Build history of the part. All positions in model axes, mm. Give positions to 0.01 mm unless a question says otherwise; leave off trailing zeros. Order: outer loops, then holes, each group sorted by start corner. A loop starts at its lowest first (then second) coordinate and runs counter-clockwise, first axis right, second up. Notation, with made-up numbers: (39.5, 25) -> (49.5, 25) arc R8 ccw to (49.5, 40) -> close; hole circle Ø8 at (42, -34.75). An arc over 180 degrees is marked (long way). One line per item, written item: value. Start each with the question number.
(1) Probe line 1 (X direction, y = 8.5, z = 122.5) (3 decimals); line 2 (X direction, y = 10.5, z = -304.8) (3 decimals). List the from-to ranges inside material, lowest first.
(2) Saw through at B-B on z = 277.5. Give the cut face in (x, y) (3 decimals).
(3) Saw through at A-A on y = 1.75. Give the cut face in (x, z) (3 decimals).
```python
from build123d import *

# Parameters (mm, degrees)
BOSS_EXTRUDE1_DEPTH             = 342.9
BOSS_EXTRUDE1_DEPTH_BACK        = 342.9
SKETCH3_W                       = 25.4
SKETCH3_H                       = 25.4
SKETCH3_W_2                     = 19.05
SKETCH3_H_2                     = 19.05
F_5_32_0_15625_DIAMETER_HOLE1_D = 3.96875
F_1_4_0_25_DIAMETER_HOLE1_D     = 6.35
F_1_4_0_25_DIAMETER_HOLE2_D     = 6.35


with BuildPart() as part:
    # Sketch3 → Boss-Extrude1 (new, two sides: drawn at the far end of the back side and taken through both)
    with BuildSketch(Plane.XY.offset(-BOSS_EXTRUDE1_DEPTH_BACK)):
        Rectangle(SKETCH3_W, SKETCH3_H)
        Rectangle(SKETCH3_W_2, SKETCH3_H_2, mode=Mode.SUBTRACT)
    extrude(amount=BOSS_EXTRUDE1_DEPTH + BOSS_EXTRUDE1_DEPTH_BACK)

    # 5/32 (0.15625) Diameter Hole1 (through all)
    with Locations(Plane(origin=(0, 12.7, 0), x_dir=(1, 0, 0), z_dir=(0, 1, 0))):
        with Locations((0, 152.4), (0, -178.5118096)):
            Hole(F_5_32_0_15625_DIAMETER_HOLE1_D / 2)

    # 1/4 (0.25) Diameter Hole1 (through all)
    with Locations(Plane(origin=(0, 12.7, 0), x_dir=(1, 0, 0), z_dir=(0, 1, 0))):
        with Locations((0, 330.2), (0, 304.8), (0, 279.4)):
            Hole(F_1_4_0_25_DIAMETER_HOLE1_D / 2)

    # 1/4 (0.25) Diameter Hole2 (through all)
    with Locations(Plane(origin=(0, 12.7, 0), x_dir=(1, 0, 0), z_dir=(0, 1, 0))):
        with Locations((0, -330.911799988), (0, -305.511799988)):
            Hole(F_1_4_0_25_DIAMETER_HOLE2_D / 2)


solid = part.part
```
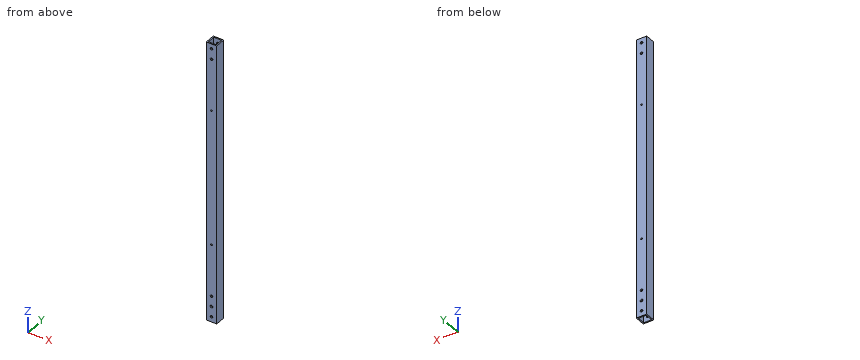
Results below:
1. line 1: x = -12.7 to -9.525, 9.525 to 12.7
1. line 2: x = -12.7 to -3.175, 3.175 to 12.7
2. outline: (-12.7, -12.7) -> (12.7, -12.7) -> (12.7, 12.7) -> (-12.7, 12.7) -> close; hole (-9.525, -9.525) -> (9.525, -9.525) -> (9.525, 9.525) -> (-9.525, 9.525) -> close
3. outline: (-12.7, -342.9) -> (-9.525, -342.9) -> (-9.525, 342.9) -> (-12.7, 342.9) -> close; (9.525, -342.9) -> (12.7, -342.9) -> (12.7, 342.9) -> (9.525, 342.9) -> close
